Geometry check sheet. Reference: drawing and pictorial views, mm from the part's lowest x, y, z. Give positions to 0.01 mm unless a question says otherwise; leave off trailing zeros. Write each loop counter-clockwise with the first axis right and the second up, starting at its lowest first coordinate (ties: lowest second). Pieces come first, ordered by that corner, then holes. Notation, with made-up numbers: (14, -1) - (40, -1) arc R14 cw to (40, 17) - close; hole circle Ø5 at (18, 87). An arc over 180 degrees is marked (long way). Write item = value, one per line. Start each with the question number.
(1) Section check C-C, the plane x = 5. Enter the section's corners in (y, z), plus the area to 3 significant figures.
(2) Section check B-B, the plane y = 15. Enter the section's corners in (x, z), plus the area to 3 significant figures.
(3) Section check A-A, the plane z = 1.1. Enter the section's corners in (x, y), plus the area to 3 significant figures.
(4) Thickness scan on L1, parallel to X at y = 5, z = 0.7; L2, parallel to X at y = 6, z = 0.8. Record the ranges inside material, lowest first.
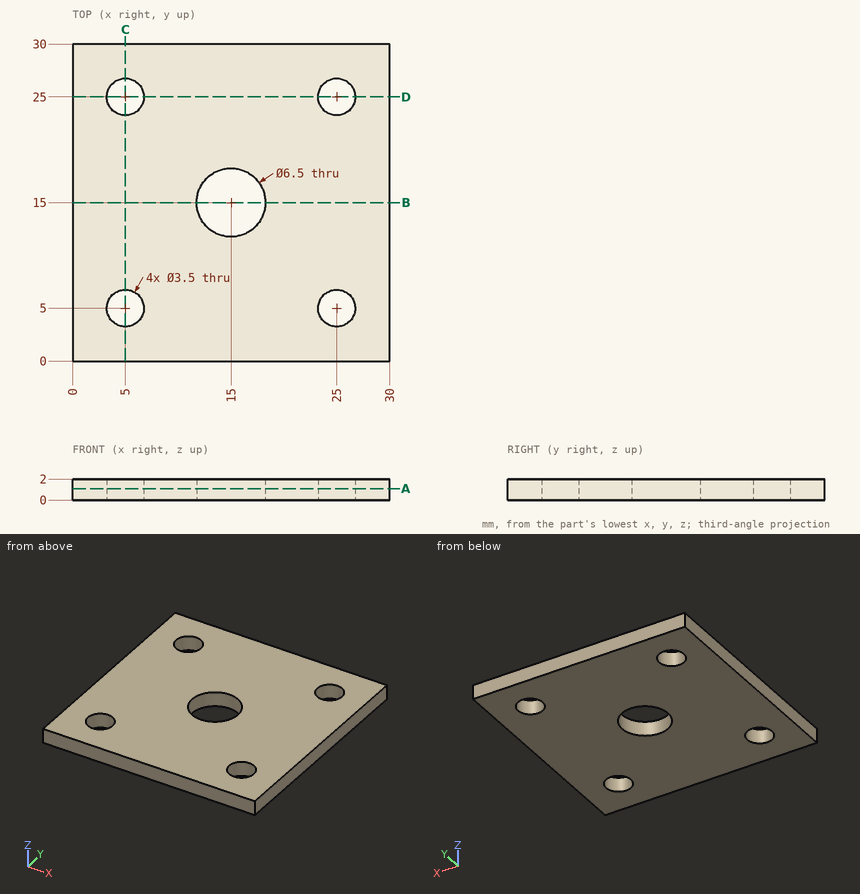
Model answer:
q1.outline = (0, 0) - (3.25, 0) - (3.25, 2) - (0, 2) - close; (6.75, 0) - (23.25, 0) - (23.25, 2) - (6.75, 2) - close; (26.75, 0) - (30, 0) - (30, 2) - (26.75, 2) - close
q1.area = 46.0 mm²
q2.outline = (0, 0) - (11.75, 0) - (11.75, 2) - (0, 2) - close; (18.25, 0) - (30, 0) - (30, 2) - (18.25, 2) - close
q2.area = 47.0 mm²
q3.outline = (0, 0) - (30, 0) - (30, 30) - (0, 30) - close; hole circle Ø3.5 at (5, 5); hole circle Ø3.5 at (5, 25); hole circle Ø6.5 at (15, 15); hole circle Ø3.5 at (25, 5); hole circle Ø3.5 at (25, 25)
q3.area = 828 mm²
q4.L1 = 0 to 3.25, 6.75 to 23.25, 26.75 to 30
q4.L2 = 0 to 3.56, 6.44 to 23.56, 26.44 to 30
